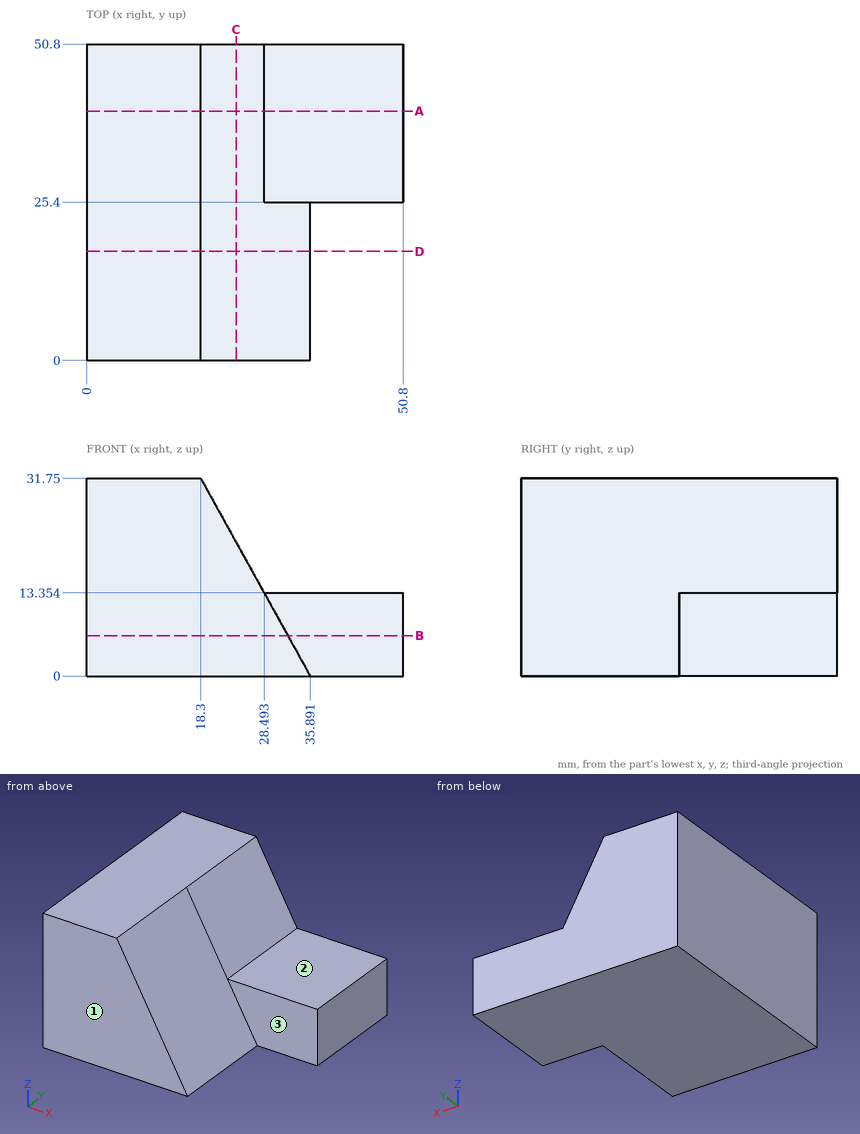
Study the drawing (mm; zero at the part's minimum x, y, z) and answer. A direction names the side the tool comes from. Give positions to 0.01 mm unless a question says otherwise; leave off trailing zeros. Loops run counter-clockwise (first coordinate to the right, second up) from the corner with the lowest first, then second, coordinate; pieces in that order, holes last. Notation, with made-up numbers: (18.25, 60.5) - (54.25, 60.5) arc R13 cw to (54.25, 81.5) - close; hole circle Ø5 at (-8.75, -31.5). An arc over 180 degrees is marked (long way). Use CSV: the item, a comma, the result in double quotes. Start each with the question number.
(1) Find section C-C, the plane x = 24. Determine the outline of the cut face in (y, z).
(2) Find section D-D, the plane y = 17.5. Determine the outline of the cut face in (x, z), plus the area to 3 significant figures.
(3) Find section A-A, the plane y = 40. Determine the outline of the cut face in (x, z).
(4) Each of these flat-tipped pins is pushed along its axis until it touches: pin 1 (5 mm diameter, centred on x = 40, z = 12, fed in from -Y); pin 2 (10 mm diameter, centred on y = 22.5, z = 25.5, fed in from +X); pin 3 (6.5 mm diameter, centred on x = 35, y = 34, fed in from +Z). Where does it stop, or does it pass through?
(5) Find the intervals of material crossed by L1, parallel to Z at x = 33, y = 36; L2, parallel to X at y = 42, z = 19.5; L3, parallel to X at y = 10.5, z = 20.5 (1 decimal), in increasing order.
(6) A tool of negligible diameter and unlimited length cuts with its end or side. For the marked faces 1, 2 and 3, from which of +Z, -Z, +X, -X, +Y, -Y can it reach the whole face along a straight path? Write none if from no direction.
(7) Find section B-B, the plane z = 6.5. Determine the outline of the cut face in (x, y).
Results found:
1,outline,"(0, 0) - (50.8, 0) - (50.8, 21.46) - (0, 21.46) - close"
2,outline,"(0, 0) - (35.89, 0) - (18.3, 31.75) - (0, 31.75) - close"
2,area,"860 mm^2"
3,outline,"(0, 0) - (50.8, 0) - (50.8, 13.35) - (28.49, 13.35) - (18.3, 31.75) - (0, 31.75) - close"
4,pin 1,"y = 25.4"
4,pin 2,"x = 24.53"
4,pin 3,"z = 13.35"
5,L1,"0 to 13.35"
5,L2,"0 to 25.09"
5,L3,"0 to 24.5"
6,face 1,"+Z, -Z, +X, -X, -Y"
6,face 2,"+Z, +X, +Y, -Y"
6,face 3,"+Z, +X, -Y"
7,outline,"(0, 0) - (32.29, 0) - (32.29, 25.4) - (50.8, 25.4) - (50.8, 50.8) - (0, 50.8) - close"
